CAD build for the part. Positions are in the model's coordinates, mm. A direction names the side the tool comes from. Give positions to 0.01 mm unless a question says otherwise; leave off trailing zeros. Order: outer loops, then holes, each group sorted by start corner. A loop starts at its lowest first (then second) coordinate and runs counter-clockwise, first axis right, second up.
Item 1: Band-saw the part on A-A on y = -0.5. Count the separate pieces of the cut face and the enclosed holes in it, plus the area to 3 significant figures.
Item 2: Band-saw the part on B-B on x = 21. Give the cut face in (y, z) (3 decimals), plus the area to 4 significant figures.
Item 3: Which spindle directions (+Z, -Z, +X, -X, +Y, -Y) get a long thin tool onto all of the face, cutting with end or side? Do faces 1 (the flat face through (16.5, 0, 22)), 2 (the cylindrical face through (39.58, -0.81, 42.74)), 3 (the flat face through (16.993, -1, 22)), 4 (the flat face through (31, -4, 40.792)), 5 (the flat face through (40, -1, 26.822)). Say none if no direction does.
Item 4: Band-saw the part on D-D on z = 29.5. Give the cut face in (x, y) (1 decimal).
Item 5: Band-saw the part on C-C on x = 32. Give the cut face in (y, z) (3 decimals), plus the area to 3 significant figures.
Item 6: Flat gauge pins, fed straight in: P1, Ø1.1, axis at x = 41.25, z = 10.16, coming from the +Y side; P2, Ø4, axis at x = 14, z = 21, coming from the +Y side; P3, Ø6, axis at x = 36.5, z = 8, coming from the -Y side; P4, Ø2, axis at y = -4, z = 35, coming from the +X side. Where does each tip first touch, or does it go through?
Item 7: Wall check: L1, parallel to Y at x = 10, z = 5.5 (3 decimals); L2, parallel to Z at x = 28.5, y = -3.35; L3, parallel to Z at x = 30, y = -2.9. Give the ranges that are in metal, low to high.
Item 8: Two-plate mould, pull along Z, no slides. Class faces 6 (the cylindrical face through (40.74, -4.14, 41.36)), 7 (the flat face through (22, -3, 43.307)), 8 (the cylindrical face through (39.577, -0.811, 0.566)): released by +Z, released by -Z, zero draft, split by the parting line, or undercut.
```python
from build123d import *

# Parameters (mm, degrees)
F0_W         = 43.307
F0_H         = 43.307
F1_DEPTH     = 1.27
F3_DEPTH     = 3.175
F5_DEPTH     = 1.905
F6_R         = 0.889
F7_DEPTH     = 5.081
F8_W         = 9.3218
F8_H         = 9.3218
F8_W_2       = 7.0612
F8_H_2       = 10.3124
F10_DEPTH    = 1.27
F11_D        = 3.175
F14_D        = 2.54
F15_R        = 6.35
F16_T4_DEPTH = 12.7851645967
F16_T9_DEPTH = 12.8907938144
F17_R        = 0.7874
F18_D        = 3.175
F18_DEPTH    = 3.175
F18_TIP      = 0.9538662327
F19_T4_DEPTH = 6.3848359064
F19_T9_DEPTH = 6.2809008493


# Not quite as in the source:
# - a fillet or chamfer that OpenCascade refuses, or shapes differently, is made with other operations: its cross-section is extruded or revolved along the edge and cut away or added


with BuildPart() as f1:
    # F0 (on Front) → F1 (new body)
    with BuildSketch(Plane.XZ):
        with Locations((21.6535, 21.6535)):
            Rectangle(F0_W, F0_H)
    extrude(amount=F1_DEPTH)

    # F2 (on Front) → F3 (join)
    with BuildSketch(Plane.XZ):
        with BuildLine():
            Line((43.307, 43.307), (0, 43.307))
            Line((0, 43.307), (0, 0))
            Line((0, 0), (43.307, 0))
            Line((43.307, 0), (43.307, 1.0922))
            Line((43.307, 1.0922), (21.6408, 1.0922))
            ThreePointArc((21.6408, 1.0922), (1.0668, 21.6662), (21.6408, 42.2402))
            Line((21.6408, 42.2402), (43.307, 42.2402))
            Line((43.307, 42.2402), (43.307, 43.307))
        make_face()
    extrude(amount=F3_DEPTH)

    # F4 (on face) → F5 (join)
    with BuildSketch(Plane.XZ.offset(3.175)):
        with BuildLine():
            Line((43.307, 43.307), (0, 43.307))
            Line((0, 43.307), (0, 0))
            Line((0, 0), (43.307, 0))
            Line((43.307, 0), (43.307, 2.54))
            Line((43.307, 2.54), (21.6408, 2.54))
            ThreePointArc((21.6408, 2.54), (2.5146, 21.6662), (21.6408, 40.7924))
            Line((21.6408, 40.7924), (43.307, 40.7924))
            Line((43.307, 40.7924), (43.307, 43.307))
        make_face()
    extrude(amount=F5_DEPTH)

    # F6 (on face) → F7 (cut, through all)
    with BuildSketch(Plane(origin=(0, 0, 0), x_dir=(-1, 0, 0), z_dir=(0, 1, 0))):
        with Locations((-41.2496, 33.1724)):
            Circle(F6_R)
        with Locations((-2.667, 33.1724)):
            Circle(F6_R)
        with Locations((-41.2496, 10.16)):
            Circle(F6_R)
        with Locations((-2.667, 10.16)):
            Circle(F6_R)
    extrude(amount=-F7_DEPTH, mode=Mode.SUBTRACT)

    # F8 (on face) → F10 (cut, through all)
    with BuildSketch(Plane.XZ.offset(1.27)):
        with Locations((21.6535, 21.6535)):
            Rectangle(F8_W, F8_H)
        with Locations((39.7764, 21.6662)):
            Rectangle(F8_W_2, F8_H_2)
    extrude(amount=-F10_DEPTH, mode=Mode.SUBTRACT)

    # F11 (through all)
    with Locations(Plane(origin=(0, 0, 0), x_dir=(-1, 0, 0), z_dir=(0, 1, 0))):
        with Locations((-4.0894, 39.2176), (-4.0894, 4.0894)):
            Hole(F11_D / 2)

    # F14 (through all)
    with Locations(Plane(origin=(0, 0, 0), x_dir=(-1, 0, 0), z_dir=(0, 1, 0))):
        with Locations((-21.6535, 32.1564), (-21.6535, 11.176)):
            Hole(F14_D / 2)

    # F15
    f15_edges = [f1.edges().sort_by_distance(p)[0] for p in [
        (0, -2.54, 43.307),
        (43.307, -2.54, 43.307),
        (43.307, -2.54, 0),
        (0, -2.54, 0),
    ]]
    fillet(f15_edges, radius=F15_R)

    # F16: fillet of radius 0.8128 on 2 edges, made by hand


with BuildPart() as f16_tool2:
    # F16_s3 → F16_t4 (new body)
    with BuildSketch(Plane.XZ.offset(10.5200822984)):
        with BuildLine():
            ThreePointArc((40.005, 2.54), (40.7835212046, 1.9607563614), (40.452412844, 1.0486238532))
            ThreePointArc((40.452412844, 1.0486238532), (41.3090658387, 1.7259300464), (42.037, 2.54))
            Line((42.037, 2.54), (40.005, 2.54))
        make_face()
    extrude(amount=-F16_T4_DEPTH)

    split(bisect_by=Plane.XZ.offset(1.27), keep=Keep.TOP)


with BuildPart() as f1_1:
    add(f1.part)

    # F16_t1: cut F16_tool2
    add(f16_tool2.part, mode=Mode.SUBTRACT)


with BuildPart() as f16_tool7:
    # F16_s8 → F16_t9 (new body)
    with BuildSketch(Plane.XZ.offset(10.5728969072)):
        with BuildLine():
            ThreePointArc((39.9661228955, 40.7924), (40.7456166441, 41.374910322), (40.4078290086, 42.2875045872))
            ThreePointArc((40.4078290086, 42.2875045872), (41.2779959557, 41.6101165847), (42.0178504068, 40.7924))
            Line((42.0178504068, 40.7924), (39.9661228955, 40.7924))
        make_face()
    extrude(amount=-F16_T9_DEPTH)

    split(bisect_by=Plane.XZ.offset(1.27), keep=Keep.TOP)


with BuildPart() as f1_2:
    add(f1_1.part)

    # F16_t6: cut F16_tool7
    add(f16_tool7.part, mode=Mode.SUBTRACT)

    # F17
    f17_edges = [f1_2.edges().sort_by_distance(p)[0] for p in [
        (43.307, -0.635, 26.8224),
        (36.2458, -0.635, 26.8224),
        (16.9926, -0.635, 26.3144),
        (16.9926, -0.635, 16.9926),
        (26.3144, -0.635, 16.9926),
        (43.307, -0.635, 16.51),
        (36.2458, -0.635, 16.51),
        (26.3144, -0.635, 26.3144),
    ]]
    fillet(f17_edges, radius=F17_R)

    # F18
    with Locations(Plane(origin=(0, 0, 0), x_dir=(-1, 0, 0), z_dir=(0, 1, 0))):
        with Locations((-39.2176, 4.0894), (-39.2176, 39.2176)):
            Hole(F18_D / 2, depth=F18_DEPTH)
            with Locations((0, 0, -(F18_DEPTH + F18_TIP / 2))):  # 118° drill point
                Cone(0, F18_D / 2, F18_TIP, mode=Mode.SUBTRACT)

    # F19: fillet of radius 0.396875 on 2 edges, made by hand


with BuildPart() as f19_tool2:
    # F19_s3 → F19_t4 (new body)
    with BuildSketch(Plane.XZ.offset(-3.2098359064)):
        with BuildLine():
            ThreePointArc((38.8580757032, 43.0157466667), (39.1315562434, 42.57697322), (38.7392584717, 42.2402))
            Line((38.7392584717, 42.2402), (38.7392584717, 42.2005125))
            Line((38.7392584717, 42.2005125), (40.4734874982, 42.2005125))
            Line((40.4734874982, 42.2005125), (40.4982611604, 42.2712058594))
            ThreePointArc((40.4982611604, 42.2712058594), (40.4293966899, 42.3208202408), (38.8699574263, 43.0536138333))
            Line((38.8699574263, 43.0536138333), (38.8580757032, 43.0157466667))
        make_face()
    extrude(amount=F19_T4_DEPTH)

    split(bisect_by=Plane.XZ.offset(1.27), keep=Keep.TOP)


with BuildPart() as f1_3:
    add(f1_2.part)

    # F19_t1: cut F19_tool2
    add(f19_tool2.part, mode=Mode.SUBTRACT)


with BuildPart() as f19_tool7:
    # F19_s8 → F19_t9 (new body)
    with BuildSketch(Plane.XZ.offset(-3.1059008493)):
        with BuildLine():
            ThreePointArc((38.9423609411, 0.3183466667), (39.2101451473, 0.7581600602), (38.8182758823, 1.0922))
            Line((38.8182758823, 1.0922), (38.8182758823, 1.1318875))
            Line((38.8182758823, 1.1318875), (40.5123646026, 1.1318875))
            Line((40.5123646026, 1.1318875), (40.5371382648, 1.0611941406))
            ThreePointArc((40.5371382648, 1.0611941406), (40.4742591743, 1.0154902523), (38.954769447, 0.2806488333))
            Line((38.954769447, 0.2806488333), (38.9423609411, 0.3183466667))
        make_face()
    extrude(amount=F19_T9_DEPTH)

    split(bisect_by=Plane.XZ.offset(1.27), keep=Keep.TOP)


with BuildPart() as f1_4:
    add(f1_3.part)

    # F19_t6: cut F19_tool7
    add(f19_tool7.part, mode=Mode.SUBTRACT)


solid = f1_4.part
```
The answers:
1. separate pieces: 1
1. enclosed holes: 11
1. area: 1,630 mm2
2. outline: (-5.08, 0) - (0, 0) - (0, 10.087) - (-1.27, 10.087) - (-1.27, 1.102) - (-3.175, 1.102) - (-3.175, 2.551) - (-5.08, 2.551) - close; (-5.08, 40.782) - (-3.175, 40.782) - (-3.175, 42.23) - (-1.27, 42.23) - (-1.27, 33.245) - (0, 33.245) - (0, 43.307) - (-5.08, 43.307) - close; (-1.27, 12.265) - (0, 12.265) - (0, 16.993) - (-1.27, 16.993) - close; (-1.27, 26.314) - (0, 26.314) - (0, 31.067) - (-1.27, 31.067) - close
2. area: 51.45 mm2
3. face 1: +Z, -Z, +X, -X, +Y
3. face 2: +Z, +X, +Y, -Y
3. face 3: +Y, -Y
3. face 4: +X, -Y
3. face 5: +X, +Y, -Y
4. outline: (0, -5.1) - (4.2, -5.1) - (4.2, -3.2) - (2.6, -3.2) - (2.6, -1.3) - (43.3, -1.3) - (43.3, 0) - (0, 0) - close
5. outline: (-5.08, 0) - (0, 0) - (0, 43.307) - (-5.08, 43.307) - (-5.08, 40.792) - (-3.175, 40.792) - (-3.175, 42.24) - (-1.27, 42.24) - (-1.27, 1.092) - (-3.175, 1.092) - (-3.175, 2.54) - (-5.08, 2.54) - close
5. area: 68.7 mm2
6. P1: passes through
6. P2: stops at y = 0
6. P3: stops at y = -1.27
6. P4: stops at x = 8.98
7. L1: y = -5.08 to -3.175, -1.27 to 0
7. L2: z = 0 to 2.54, 40.79 to 43.31
7. L3: z = 0 to 1.09, 42.24 to 43.31
8. face 6: undercut
8. face 7: released by +Z
8. face 8: released by -Z
